Check sheet for the modelled part. Datum: model origin and axes. Units: mm. A direction names the side the tool comes from. Coordinates: 2 decimals unless noted, no trailing zeros. Loops run counter-clockwise (first coordinate to the right, second up) from the corner with the lowest first, then second, coordinate; pieces in that order, holes last. Notation, with made-up numbers: (-30, 28) -> (-23, 28) arc R21 ccw to (-23, 58) -> close; hole circle Ø9 at (78.5, 20). An arc over 180 degrees is marked (long way). Use CSV: the item, a comma, the result in double quotes.
```python
from build123d import *

# Parameters (mm, degrees)
BOSS_EXTRUDE1_DEPTH = 10
BOSS_EXTRUDE2_DEPTH = 0.8
FILLET1_R           = 10
SKETCH3_R           = 1.65
BOSS_EXTRUDE4_DEPTH = 4
SKETCH4_R           = 2.8
CUT_EXTRUDE1_DEPTH  = 7


with BuildPart() as part:
    # Sketch1 → Boss-Extrude1 (new body)
    with BuildSketch(Plane.XY):
        with BuildLine():
            Line((-7.6, -4.13067791), (-7.6, -9.5))
            Line((-7.6, -9.5), (-10.1, -9.5))
            Line((-10.1, -9.5), (-10.1, -6.479969136))
            ThreePointArc((-10.1, -6.479969136), (0, 12), (10.1, -6.479969136))
            Line((10.1, -6.479969136), (10.1, -9.5))
            Line((10.1, -9.5), (7.6, -9.5))
            Line((7.6, -9.5), (7.6, -4.13067791))
            ThreePointArc((7.6, -4.13067791), (0, 8.65), (-7.6, -4.13067791))
        make_face()
    extrude(amount=BOSS_EXTRUDE1_DEPTH)

    # Sketch2 → Boss-Extrude2 (add)
    with BuildSketch(Plane.XY.offset(10)):
        with BuildLine():
            Line((7.6, -4.13067791), (7.6, -9.5))
            Line((7.6, -9.5), (-7.6, -9.5))
            Line((-7.6, -9.5), (-7.6, -4.13067791))
            ThreePointArc((-7.6, -4.13067791), (0, 8.65), (7.6, -4.13067791))
        make_face()
    extrude(amount=-BOSS_EXTRUDE2_DEPTH)

    # Fillet1
    fillet1_edges = [part.edges().sort_by_distance(p)[0] for p in [
        (10.1, -6.479969136, 5),
        (-10.1, -6.479969136, 5),
    ]]
    fillet(fillet1_edges, radius=FILLET1_R)

    # Sketch3 → Boss-Extrude4 (add)
    with BuildSketch(Plane(origin=(0, 0, 0), x_dir=(-1, 0, 0), z_dir=(0, 0, -1))):
        with BuildLine():
            ThreePointArc((14, 3.15), (17.15, 0), (14, -3.15))
            ThreePointArc((14, -3.15), (12.130662272, -3.6913019), (10.839796225, -5.147700243))
            ThreePointArc((10.839796225, -5.147700243), (12, 0), (10.839796225, 5.147700243))
            ThreePointArc((10.839796225, 5.147700243), (12.130662272, 3.6913019), (14, 3.15))
        make_face()
        with Locations((14, 0)):
            Circle(SKETCH3_R, mode=Mode.SUBTRACT)
        with BuildLine():
            ThreePointArc((-10.839796225, 5.147700243), (-12, 0), (-10.839796225, -5.147700243))
            ThreePointArc((-10.839796225, -5.147700243), (-12.130662272, -3.6913019), (-14, -3.15))
            ThreePointArc((-14, -3.15), (-17.15, 0), (-14, 3.15))
            ThreePointArc((-14, 3.15), (-12.130662272, 3.6913019), (-10.839796225, 5.147700243))
        make_face()
        with Locations((-14, 0)):
            Circle(SKETCH3_R, mode=Mode.SUBTRACT)
    extrude(amount=-BOSS_EXTRUDE4_DEPTH)

    # Sketch4 → Cut-Extrude1 (cut, through all)
    with BuildSketch(Plane.XY.offset(4)):
        with Locations((-14, 0)):
            Circle(SKETCH4_R)
        with Locations((14, 0)):
            Circle(SKETCH4_R)
    extrude(amount=CUT_EXTRUDE1_DEPTH, mode=Mode.SUBTRACT)


solid = part.part
```
1) Cross-section at C-C on x = 0. Record the boundary of the cut face in (y, z).
Answer below:
outline,"(-9.5, 9.2) -> (8.65, 9.2) -> (8.65, 0) -> (12, 0) -> (12, 10) -> (-9.5, 10) -> close"
2) Thickness scan on line 1 along Y through (x, z) = (-14, 0.9); line 2 along X through (y, z) = (0, 7); line 3 along Z through (x, y) = (7, 2.5). Record the ranges inside material, lowest first. Write a range as from..to.
Answer below:
line 1,"y = -3.15..-1.65, 1.65..3.15"
line 2,"x = -11.2..-8.65, 8.65..11.2"
line 3,"z = 9.2..10"
3) Access from +Z, -Z, +X, -X, +Y, -Y to the whole of each face (thin tool, end or side, straight path). Record for faces 1 (the cylindrical face through (0.25, 8.646, 4.536)), 2 (the cylindrical face through (-11.51, -3.4, 6.96)), 3 (the cylindrical face through (11.522, -3.352, 6.958)), 4 (the cylindrical face through (11.2, 0, 7)), 5 (the flat face through (-7.6, -7, 5)).
Answer below:
face 1,"-Z"
face 2,"+Z, -X, -Y"
face 3,"+Z, +X, -Y"
face 4,"+Z, +X"
face 5,"-Z, -Y"
4) Cross-section at D-D on x = -13. Record the boundary of the cut face in (y, z), and give its area (3 significant figures).
Answer below:
outline,"(-3.3, 0) -> (-1.31, 0) -> (-1.31, 4) -> (-3.3, 4) -> close; (1.31, 0) -> (3.3, 0) -> (3.3, 4) -> (1.31, 4) -> close"
area,"15.9 mm²"
5) Go/stop test with flat-tipped pins: pin 1 Ø4 at (y, z) = (-5, 8) entering from +X; pin 2 Ø10 at (x, y) = (-13, 3) entering from -Z; pin 3 Ø2.5 at (y, z) = (-7.5, 4) entering from -X; pin 4 Ø0.6 at (y, z) = (-9, 6) entering from -X. Record where each tip stops, or that it passes through.
Answer below:
pin 1,"stops at x = 11.62"
pin 2,"stops at z = 0"
pin 3,"stops at x = -10.47"
pin 4,"stops at x = -10.1"
6) Cross-section at B-B on z = 3.5. Record the boundary of the cut face in (x, y), and give its area (3 significant figures).
Answer below:
outline,"(-14, -3.15) arc R3.5 cw to (-10.89, -5.04) arc R10 cw to (-10.1, -8.94) -> (-10.1, -9.5) -> (-7.6, -9.5) -> (-7.6, -4.13) arc R8.65 cw (long way) to (7.6, -4.13) -> (7.6, -9.5) -> (10.1, -9.5) -> (10.1, -8.94) arc R10 cw to (10.89, -5.04) arc R3.5 cw to (14, -3.15) arc R3.15 ccw to (14, 3.15) arc R3.5 cw to (10.84, 5.15) arc R12 ccw to (-10.84, 5.15) arc R3.5 cw to (-14, 3.15) arc R3.15 ccw to start; hole circle Ø3.3 at (-14, 0); hole circle Ø3.3 at (14, 0)"
area,"213 mm²"
7) Cross-section at A-A on y = 0. Record the boundary of the cut face in (x, z), and give its area (3 significant figures).
Answer below:
outline,"(-17.15, 0) -> (-15.65, 0) -> (-15.65, 4) -> (-17.15, 4) -> close; (-12.35, 0) -> (-8.65, 0) -> (-8.65, 9.2) -> (8.65, 9.2) -> (8.65, 0) -> (12.35, 0) -> (12.35, 4) -> (11.2, 4) -> (11.2, 10) -> (-11.2, 10) -> (-11.2, 4) -> (-12.35, 4) -> close; (15.65, 0) -> (17.15, 0) -> (17.15, 4) -> (15.65, 4) -> close"
area,"86.0 mm²"
